from build123d import *

# Parameters (mm, degrees)
SKETCH1_W           = 88.9
SKETCH1_H           = 101.6
BASE_EXTRUDE_DEPTH  = 2.54
WALL_EXTRUDE_DEPTH  = 2.54
CUT_EXTRUDE1_REACH  = 139.864
SKETCH3_R           = 3.4925
FILLET2_R           = 5.08
SKETCH4_R           = 2.032
CUT_EXTRUDE2_DEPTH  = 138.371503752
SKETCH5_W           = 2.54
SKETCH5_H           = 2.54
SKETCH5_W_2         = 5.08
SKETCH5_W_3         = 5.588
BOSS_EXTRUDE1_DEPTH = 12.7


with BuildPart() as part:
    # Sketch1 → Base Extrude (new body)
    with BuildSketch(Plane(origin=(0, 0, 0), x_dir=(1, 0, 0), z_dir=(0, 1, 0))):
        with Locations((44.45, 50.8)):
            Rectangle(SKETCH1_W, SKETCH1_H)
    extrude(amount=BASE_EXTRUDE_DEPTH)

    # Sketch2 → Wall Extrude (add)
    with BuildSketch(Plane(origin=(88.9, 0, 0), x_dir=(0, 0, -1), z_dir=(1, 0, 0))):
        with BuildLine():
            Line((101.6, 2.54), (101.6, 0))
            Line((101.6, 0), (0, 0))
            Line((0, 0), (0, 2.54))
            ThreePointArc((0, 2.54), (50.8, 27.94), (101.6, 2.54))
        make_face()
    wall_extrude = extrude(amount=-WALL_EXTRUDE_DEPTH)

    # Wall Mirror: Wall Extrude across plane
    add(wall_extrude.mirror(Plane(origin=(44.45, 0, 0), x_dir=(0, 0, 1), z_dir=(1, 0, 0))))

    # Sketch3 → Cut-Extrude1 (cut, up to next)
    with BuildSketch(Plane.ZY, mode=Mode.PRIVATE) as cut_extrude1_sk1:
        with Locations((-50.8, 21.2725)):
            Circle(SKETCH3_R)
    cut_extrude1_tool1 = extrude(cut_extrude1_sk1.sketch, amount=-CUT_EXTRUDE1_REACH, mode=Mode.PRIVATE) & part.part
    add(cut_extrude1_tool1.solids().sort_by_distance((0, 21.2725, -50.8))[0], mode=Mode.SUBTRACT)

    # Fillet2
    # the kernel refuses this fillet: 5.08 mm, written as the material it adds along each edge
    with BuildSketch(Plane(origin=(86.36, 2.54, -101.6), x_dir=(-1, 0, 0), z_dir=(0, 0, 1))) as fillet2_piece_1_section:
        with BuildLine():
            CenterArc((FILLET2_R, -FILLET2_R), FILLET2_R, 90, 90)
            Line((0, -FILLET2_R), (0, 0))
            Line((0, 0), (FILLET2_R, 0))
        make_face()
    fillet2_piece_1 = extrude(amount=101.6, mode=Mode.PRIVATE)
    fillet2_piece_1 = fillet2_piece_1 & Plane(origin=(85.198656014, -35.56, -50.8), x_dir=(0, 0.6000000000000003, 0.7999999999999998), z_dir=(1, 0, 0)) * Cylinder(63.5, 224, mode=Mode.PRIVATE)
    add(fillet2_piece_1)
    with BuildSketch(Plane(origin=(2.54, 2.54, -101.6), x_dir=(1, 0, 0), z_dir=(0, 0, 1))) as fillet2_piece_2_section:
        with BuildLine():
            CenterArc((FILLET2_R, FILLET2_R), FILLET2_R, 180, 90)
            Line((0, FILLET2_R), (0, 0))
            Line((0, 0), (FILLET2_R, 0))
        make_face()
    fillet2_piece_2 = extrude(amount=101.6, mode=Mode.PRIVATE)
    fillet2_piece_2 = fillet2_piece_2 & Plane(origin=(3.701343986, -35.56, -50.8), x_dir=(0, 0.6000000000000003, 0.7999999999999998), z_dir=(-1, 0, 0)) * Cylinder(63.5, 224, mode=Mode.PRIVATE)
    add(fillet2_piece_2)

    # Sketch4 → Cut-Extrude2 (cut, through all)
    with BuildSketch(Plane(origin=(0, 2.54, 0), x_dir=(1, 0, 0), z_dir=(0, 1, 0))):
        with Locations(Location((44.45, 57.15, 0), (0, 0, 270))):
            Circle(SKETCH4_R)
        with Locations(Location((44.45, 15.15, 0), (0, 0, 270))):
            Circle(SKETCH4_R)
        with Locations(Location((58.42, 74.93, 0), (0, 0, 270))):
            Circle(SKETCH4_R)
        with Locations(Location((58.42, 95.25, 0), (0, 0, 270))):
            Circle(SKETCH4_R)
        with Locations(Location((30.48, 74.93, 0), (0, 0, 90))):
            Circle(SKETCH4_R)
        with Locations(Location((30.48, 95.25, 0), (0, 0, 90))):
            Circle(SKETCH4_R)
    extrude(amount=-CUT_EXTRUDE2_DEPTH, mode=Mode.SUBTRACT)

    # Sketch5 → Boss-Extrude1 (add)
    with BuildSketch(Plane(origin=(0, 2.54, 0), x_dir=(1, 0, 0), z_dir=(0, 1, 0))):
        with Locations((87.63, 50.8)):
            Rectangle(SKETCH5_W, SKETCH5_H)
        Polygon((13.208, 82.55), (13.208, 19.05), (7.62, 19.05), (7.62, 16.51), (15.748, 16.51), (15.748, 85.09), (7.62, 85.09), (7.62, 82.55), align=None)
        with Locations((5.08, 17.78)):
            Rectangle(SKETCH5_W_2, SKETCH5_H)
        with Locations((5.08, 83.82)):
            Rectangle(SKETCH5_W_2, SKETCH5_H)
        Polygon((81.28, 83.82), (81.28, 86.36), (73.152, 86.36), (73.152, 52.07), (75.692, 52.07), (75.692, 83.82), align=None)
        Polygon((75.692, 49.53), (73.152, 49.53), (73.152, 15.24), (81.28, 15.24), (81.28, 17.78), (75.692, 17.78), align=None)
        with Locations((83.82, 50.8)):
            Rectangle(SKETCH5_W_2, SKETCH5_H)
        with Locations((78.486, 50.8)):
            Rectangle(SKETCH5_W_3, SKETCH5_H)
        with Locations((74.422, 50.8)):
            Rectangle(SKETCH5_W, SKETCH5_H)
        with Locations((83.82, 85.09)):
            Rectangle(SKETCH5_W_2, SKETCH5_H)
        with Locations((83.82, 16.51)):
            Rectangle(SKETCH5_W_2, SKETCH5_H)
    extrude(amount=BOSS_EXTRUDE1_DEPTH)


solid = part.part
Here's how the part is built. I have some questions about the finished solid (model axes, mm). A direction names the side the tool comes from. Give positions to 0.01 mm unless a question says otherwise; leave off trailing zeros. Loops run counter-clockwise (first coordinate to the right, second up) from the corner with the lowest first, then second, coordinate; pieces in that order, holes last. Notation, with made-up numbers: (-1, -16) -> (32, -16) arc R13 cw to (32, -11) -> close; hole circle Ø8 at (80, -22.75). An arc over 180 degrees is marked (long way). One line per item, written item: value.
Q1. Suppose I cut it at B-B on y = 20. Please give me the cut outline in (x, z).
Answers follow:
outline: (0, -81.55) -> (2.54, -81.55) -> (2.54, -54.05) -> (0, -54.05) -> close; (0, -47.55) -> (2.54, -47.55) -> (2.54, -20.05) -> (0, -20.05) -> close; (86.36, -81.55) -> (88.9, -81.55) -> (88.9, -20.05) -> (86.36, -20.05) -> close
Q2. On a 3-axis mill with a long thin cutter (end or side, diameter ignored), from which of +Z, -Z, +X, -X, +Y, -Y can I reach the whole of each face in a straight line? I mean faces 4 (the face through (9, 9, -16.51)), 5 (the face through (73.152, 9, -51)), 6 (the face through (3.989, 4.068, -51.244)), 7 (the face through (1.252, 17.863, -51.557)). Say none if no direction works.
Answers follow:
face 4: +Z, +Y
face 5: +Z, -Z, +Y
face 6: +Y
face 7: -X
Q3. Suppose I cut it at A-A on x = 30.48. Please give me the cut outline in (y, z).
Answers follow:
outline: (0, -101.6) -> (2.54, -101.6) -> (2.54, -97.28) -> (0, -97.28) -> close; (0, -93.22) -> (2.54, -93.22) -> (2.54, -76.96) -> (0, -76.96) -> close; (0, -72.9) -> (2.54, -72.9) -> (2.54, 0) -> (0, 0) -> close
Q4. I'm going to push flat-ended pins straight in: pin 1 Ø14 at (x, y) = (7.5, 10) entering from +Z; pin 2 Ø3 at (x, z) = (78.5, -26) entering from +Y; pin 3 Ø11.5 at (x, y) = (7, 9.5) entering from +Z; pin 4 Ø2.5 at (x, z) = (44.45, -15.15) entering from -Y. Where does each tip first touch, or does it pass through?
Answers follow:
pin 1: z = -0.95
pin 2: y = 2.54
pin 3: z = -2.15
pin 4: through
Q5. Suppose I cut it at C-C on y = 9.5. Please give me the cut outline in (x, z).
Answers follow:
outline: (0, -95.54) -> (2.54, -95.54) -> (2.54, -85.09) -> (15.75, -85.09) -> (15.75, -16.51) -> (2.54, -16.51) -> (2.54, -6.06) -> (0, -6.06) -> close; (73.15, -86.36) -> (86.36, -86.36) -> (86.36, -95.54) -> (88.9, -95.54) -> (88.9, -6.06) -> (86.36, -6.06) -> (86.36, -15.24) -> (73.15, -15.24) -> close; hole (2.54, -82.55) -> (13.21, -82.55) -> (13.21, -19.05) -> (2.54, -19.05) -> close; hole (75.69, -83.82) -> (86.36, -83.82) -> (86.36, -52.07) -> (75.69, -52.07) -> close; hole (75.69, -49.53) -> (86.36, -49.53) -> (86.36, -17.78) -> (75.69, -17.78) -> close
Q6. We'd pull the mould along Z, two halves only. Please class faces 1 (the face through (84.832, 3.989, -33.877)), 2 (the face through (80, 9, -15.24)), 3 (the face through (44, 2.54, -52)): pulls with the +Z half, pulls with the -Z half, needs draft (parallel to the pull), parting line crosses it, or undercut.
Answers follow:
face 1: undercut
face 2: pulls with the +Z half
face 3: needs draft
Q7. Suppose I cut it at D-D on z = -33. Please give me the cut outline in (x, y), then the cut area to 3 significant figures.
Answers follow:
outline: (0, 0) -> (88.9, 0) -> (88.9, 25.39) -> (86.36, 25.39) -> (86.36, 7.62) arc R5.08 cw to (81.28, 2.54) -> (75.69, 2.54) -> (75.69, 15.24) -> (73.15, 15.24) -> (73.15, 2.54) -> (15.75, 2.54) -> (15.75, 15.24) -> (13.21, 15.24) -> (13.21, 2.54) -> (7.62, 2.54) arc R5.08 cw to (2.54, 7.62) -> (2.54, 25.39) -> (0, 25.39) -> close
area: 417 mm^2
Q8. If I drill on line 1 along X through (y, z) = (13.75, -57); line 2 along X through (y, z) = (1.4, -74.93); line 3 along X through (y, z) = (13.75, -85.5), over which ranges is the centre line in solid material (lowest first)?
Answers follow:
line 1: 0 to 2.54, 13.21 to 15.75, 73.15 to 75.69, 86.36 to 88.9
line 2: 0 to 28.45, 32.51 to 56.39, 60.45 to 88.9
line 3: 0 to 2.54, 73.15 to 88.9
